Could you check a few things on this model? Use its own coordinates, in mm. Face numbers are marked on the shaded views. Give positions to 0.01 mm unless a question says otherwise; leave off trailing zeros. Order: outer loops, then holes, each group sorted by start corner. A loop starts at its lowest first (then second) coordinate and runs counter-clockwise, first axis right, second up. Notation, with made-up numbers: M 43.5,48.25 L 71.5,48.25 A29 cw 71.5,87.25 Z; hole C 63.25,24.25 d4. An arc over 180 degrees is marked long. Use a Markdown table: item, result. Add a question column.
```python
from build123d import *
from build123d.topology import SkipClean

# Parameters (mm, degrees)
SKETCH_1_R               = 18
EXTRUDE_1_DEPTH          = 1.5
EXTRUDE_2_DEPTH          = 6
EXTRUDE_2_DEPTH_BACK     = 6.5
SKETCH_2_R               = 20
SKETCH_2_R_2             = 18
CUT_EXTRUDE_START        = 1.5
SKETCH_6_R               = 1
CUT_EXTRUDE_4_DEPTH      = 8
CUT_EXTRUDE_5_DEPTH      = 30.393876913
CUT_EXTRUDE_5_DEPTH_BACK = 30.393876913
CUT_EXTRUDE_6_DEPTH      = 1.5
EXTRUDE_START            = 8
EXTRUDE_3_DEPTH          = 6.5
EXTRUDE_START_2          = 1.5
SKETCH_10_R              = 2.5
SKETCH_10_R_2            = 1.6
EXTRUDE_4_DEPTH          = 1.5


with BuildPart() as part:
    # 草图1 → 凸台-拉伸1 (new body)
    with BuildSketch(Plane(origin=(0, 0, 0), x_dir=(1, 0, 0), z_dir=(0, 1, 0))):
        with Locations(Location((0, 0, 0), (0, 0, 270))):
            Circle(SKETCH_1_R)
    extrude(amount=EXTRUDE_1_DEPTH)

    # 草图2 → 凸台-拉伸2 (add, two sides: drawn at the far end of the back side and taken through both)
    with BuildSketch(Plane(origin=(0, 0, 0), x_dir=(1, 0, 0), z_dir=(0, 1, 0)).offset(-EXTRUDE_2_DEPTH_BACK)):
        with Locations(Location((0, 0, 0), (0, 0, 270))):
            Circle(SKETCH_2_R)
        with Locations(Location((0, 0, 0), (0, 0, 270))):
            Circle(SKETCH_2_R_2, mode=Mode.SUBTRACT)
    extrude(amount=EXTRUDE_2_DEPTH + EXTRUDE_2_DEPTH_BACK)

    # 扫描2: sweep along a curve in space
    with SkipClean():  # the faces are left unmerged after this step: merging them gives an invalid solid
        with BuildLine() as sweep_2_path:
            ThreePointArc((0, 6, 18), (12.727922061, 6, 12.727922061), (18, 6, 0))
            ThreePointArc((18, 6, 0), (12.727922061, 6, -12.727922061), (0, 6, -18))
            ThreePointArc((0, 6, -18), (-12.727922061, 6, -12.727922061), (-18, 6, 0))
            ThreePointArc((-18, 6, 0), (-12.727922061, 6, 12.727922061), (0, 6, 18))
        # 草图5 → 扫描2 (sweep)
        with BuildSketch(Plane.XY):
            Polygon((-20, 6), (-18, 6), (-18, 8), align=None)
        sweep(path=sweep_2_path.line)

    # 草图6 → 切除-拉伸4 (cut)
    with SkipClean():  # the faces are left unmerged after this step: merging them gives an invalid solid
        with BuildSketch(Plane(origin=(0, 0, 0), x_dir=(1, 0, 0), z_dir=(0, 1, 0)).offset(CUT_EXTRUDE_START)):
            with Locations(Location((0, -12.5, 0), (0, 0, 270))):
                Circle(SKETCH_6_R)
            with Locations(Location((0, 12.5, 0), (0, 0, 270))):
                Circle(SKETCH_6_R)
        extrude(amount=-CUT_EXTRUDE_4_DEPTH, mode=Mode.SUBTRACT)

    # 草图7 → 切除-拉伸5 (cut, two sides: drawn at the far end of the back side and taken through both)
    with BuildSketch(Plane(origin=(0, 0, 0), x_dir=(1, 0, 0), z_dir=(0, 1, 0)).offset(-CUT_EXTRUDE_5_DEPTH_BACK)):
        with BuildLine():
            Line((-19.843134833, -2.5), (-15.07554347, -2.5))
            Line((-15.07554347, -2.5), (-15.07554347, 2.5))
            Line((-15.07554347, 2.5), (-19.843134833, 2.5))
            ThreePointArc((-19.843134833, 2.5), (-20, 0), (-19.843134833, -2.5))
        make_face()
        with BuildLine():
            Line((15.07554347, 2.5), (15.07554347, -2.5))
            Line((15.07554347, -2.5), (19.843134833, -2.5))
            ThreePointArc((19.843134833, -2.5), (20, 0), (19.843134833, 2.5))
            Line((19.843134833, 2.5), (15.07554347, 2.5))
        make_face()
    extrude(amount=CUT_EXTRUDE_5_DEPTH + CUT_EXTRUDE_5_DEPTH_BACK, mode=Mode.SUBTRACT)

    # 草图8 → 切除-拉伸6 (cut)
    with SkipClean():  # the faces are left unmerged after this step: merging them gives an invalid solid
        with BuildSketch(Plane(origin=(0, 0, 0), x_dir=(1, 0, 0), z_dir=(0, 1, 0)).offset(CUT_EXTRUDE_START)):
            with BuildLine():
                Line((10.606601706, 12.020815293), (12.001158233, 13.41537182))
                ThreePointArc((12.001158233, 13.41537182), (12.727922049, 12.727922074), (13.415371797, 12.001158259))
                Line((13.415371797, 12.001158259), (12.020815268, 10.606601731))
                ThreePointArc((12.020815268, 10.606601731), (10.606601706, 10.606601706), (10.606601706, 12.020815293))
            make_face()
            with BuildLine():
                Line((12.020815268, -10.606601731), (13.415371797, -12.001158259))
                ThreePointArc((13.415371797, -12.001158259), (12.727922049, -12.727922074), (12.001158233, -13.41537182))
                Line((12.001158233, -13.41537182), (10.606601706, -12.020815293))
                ThreePointArc((10.606601706, -12.020815293), (10.606601706, -10.606601706), (12.020815268, -10.606601731))
            make_face()
            with BuildLine():
                Line((-10.606601706, -12.020815293), (-12.001158233, -13.41537182))
                ThreePointArc((-12.001158233, -13.41537182), (-12.727922049, -12.727922074), (-13.415371797, -12.001158259))
                Line((-13.415371797, -12.001158259), (-12.020815268, -10.606601731))
                ThreePointArc((-12.020815268, -10.606601731), (-10.606601706, -10.606601706), (-10.606601706, -12.020815293))
            make_face()
            with BuildLine():
                Line((-12.020815268, 10.606601731), (-13.415371797, 12.001158259))
                ThreePointArc((-13.415371797, 12.001158259), (-12.727922049, 12.727922074), (-12.001158233, 13.41537182))
                Line((-12.001158233, 13.41537182), (-10.606601706, 12.020815293))
                ThreePointArc((-10.606601706, 12.020815293), (-10.606601706, 10.606601706), (-12.020815268, 10.606601731))
            make_face()
        extrude(amount=-CUT_EXTRUDE_6_DEPTH, mode=Mode.SUBTRACT)

    # 草图9 → 凸台-拉伸3 (add)
    with SkipClean():  # the faces are left unmerged after this step: merging them gives an invalid solid
        with BuildSketch(Plane(origin=(0, 0, 0), x_dir=(1, 0, 0), z_dir=(0, 1, 0)).offset(EXTRUDE_START)):
            with BuildLine():
                Line((12.020815268, -10.606601731), (13.415371797, -12.001158259))
                ThreePointArc((13.415371797, -12.001158259), (13.906042657, -11.428997228), (14.372329608, -10.836795727))
                Line((14.372329608, -10.836795727), (13.081475446, -9.545941553))
                ThreePointArc((13.081475446, -9.545941553), (9.545941558, -9.545941548), (9.545941537, -13.081475443))
                Line((9.545941537, -13.081475443), (10.8367957, -14.372329629))
                ThreePointArc((10.8367957, -14.372329629), (11.428997201, -13.906042679), (12.001158233, -13.41537182))
                Line((12.001158233, -13.41537182), (10.606601718, -12.020815281))
                ThreePointArc((10.606601718, -12.020815281), (10.606601731, -10.606601731), (12.020815268, -10.606601731))
            make_face()
            with BuildLine():
                Line((-10.606601718, -12.020815281), (-12.001158233, -13.41537182))
                ThreePointArc((-12.001158233, -13.41537182), (-11.428997201, -13.906042679), (-10.8367957, -14.372329629))
                Line((-10.8367957, -14.372329629), (-9.545941547, -13.081475453))
                ThreePointArc((-9.545941547, -13.081475453), (-9.545941551, -9.545941542), (-13.081475462, -9.545941556))
                Line((-13.081475462, -9.545941556), (-14.372329609, -10.836795726))
                ThreePointArc((-14.372329609, -10.836795726), (-13.906042657, -11.428997227), (-13.415371797, -12.001158259))
                Line((-13.415371797, -12.001158259), (-12.020815281, -10.606601718))
                ThreePointArc((-12.020815281, -10.606601718), (-10.606601718, -10.606601718), (-10.606601718, -12.020815281))
            make_face()
            with BuildLine():
                Line((10.606601718, 12.020815281), (12.001158233, 13.41537182))
                ThreePointArc((12.001158233, 13.41537182), (11.428997201, 13.906042679), (10.8367957, 14.372329629))
                Line((10.8367957, 14.372329629), (9.545941547, 13.081475453))
                ThreePointArc((9.545941547, 13.081475453), (9.545941551, 9.545941542), (13.081475462, 9.545941556))
                Line((13.081475462, 9.545941556), (14.372329609, 10.836795726))
                ThreePointArc((14.372329609, 10.836795726), (13.906042657, 11.428997227), (13.415371797, 12.001158259))
                Line((13.415371797, 12.001158259), (12.020815281, 10.606601718))
                ThreePointArc((12.020815281, 10.606601718), (10.606601718, 10.606601718), (10.606601718, 12.020815281))
            make_face()
            with BuildLine():
                Line((-12.020815268, 10.606601731), (-13.415371797, 12.001158259))
                ThreePointArc((-13.415371797, 12.001158259), (-13.906042657, 11.428997228), (-14.372329608, 10.836795727))
                Line((-14.372329608, 10.836795727), (-13.081475446, 9.545941553))
                ThreePointArc((-13.081475446, 9.545941553), (-9.545941558, 9.545941548), (-9.545941537, 13.081475443))
                Line((-9.545941537, 13.081475443), (-10.8367957, 14.372329629))
                ThreePointArc((-10.8367957, 14.372329629), (-11.428997201, 13.906042679), (-12.001158233, 13.41537182))
                Line((-12.001158233, 13.41537182), (-10.606601718, 12.020815281))
                ThreePointArc((-10.606601718, 12.020815281), (-10.606601731, 10.606601731), (-12.020815268, 10.606601731))
            make_face()
        extrude(amount=-EXTRUDE_3_DEPTH)

    # 草图10 → 凸台-拉伸4 (add)
    # profile 1 of 2: a face of its own
    with SkipClean():  # the faces are left unmerged after this step: merging them gives an invalid solid
        with BuildSketch(Plane(origin=(0, 0, 0), x_dir=(1, 0, 0), z_dir=(0, 1, 0)).offset(EXTRUDE_START_2)):
            with Locations(Location((0, 12.5, 0), (0, 0, 270))):
                Circle(SKETCH_10_R)
            with Locations(Location((0, 12.5, 0), (0, 0, 270))):
                Circle(SKETCH_10_R_2, mode=Mode.SUBTRACT)
        # profile 2 of 2: a face of its own
        with BuildSketch(Plane(origin=(0, 0, 0), x_dir=(1, 0, 0), z_dir=(0, 1, 0)).offset(EXTRUDE_START_2)):
            with Locations(Location((0, -12.5, 0), (0, 0, 270))):
                Circle(SKETCH_10_R)
            with Locations(Location((0, -12.5, 0), (0, 0, 270))):
                Circle(SKETCH_10_R_2, mode=Mode.SUBTRACT)
        extrude(amount=EXTRUDE_4_DEPTH)


solid = part.part
```
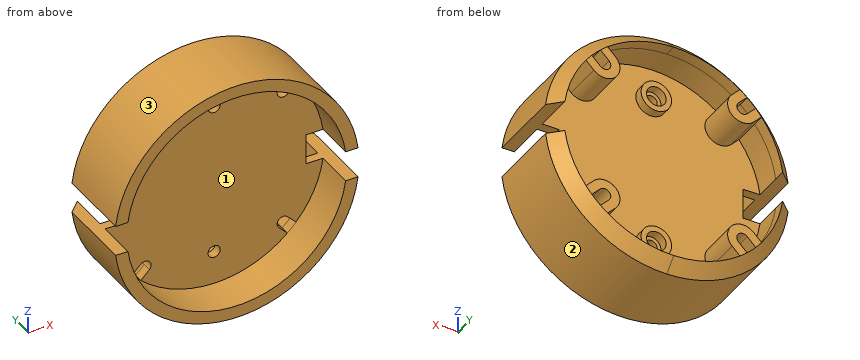
1) We'd pull the mould along Z, two halves only. Please class the marked faces 1, 2 and 3: pulls with the +Z half, pulls with the -Z half, needs draft (parallel to the pull), parting line crosses it, or undercut.
2) Suppose I cut it at C-C on z = -2. Please give me the cut outline in (x, y), and give its area (3 significant figures).
3) Please list where these lines run through material, in increasing order: line 1 (X direction, y = 2.6, z = -12.5); line 2 (Y direction, x = -7.5, z = 1); line 3 (X direction, y = 6.5, z = -8). Write a range as from..to.
4) Suppose I cut it at B-B on y = 5.5. Count the separate pieces of the cut face and the enclosed holes in it, and give its area (3 significant figures).
5) For pin 1 (10.5 mm diameter, centred on x = 1.5, z = -3, fed in from -Y); pin 2 (3 mm diameter, centred on x = 2.5, y = -2.5, fed in from -Z) (3 decimals); pin 3 (1.2 mm diameter, centred on y = 0.5, z = 0, fed in from -X), each with a flat end and sliding along its axis, tell me the tip position at first contact or that it passes through.
Values found:
| question | item | result |
|---|---|---|
| 1 | face 1 | undercut |
| 1 | face 2 | pulls with the -Z half |
| 1 | face 3 | pulls with the +Z half |
| 2 | outline | M -15.08,0 L 15.08,0 L 15.08,1.5 L -15.08,1.5 Z |
| 2 | area | 45.2 mm^2 |
| 3 | line 1 | x = -15.61..-12.95, -11.09..-9.11, -2.5..-1.6, 1.6..2.5, 9.11..11.09, 12.95..15.61 |
| 3 | line 2 | y = 0..1.5 |
| 3 | line 3 | x = -17.78..-16.12, 16.12..17.78 |
| 4 | separate pieces | 2 |
| 4 | enclosed holes | 4 |
| 4 | area | 275 mm^2 |
| 5 | pin 1 | stops at y = 0 |
| 5 | pin 2 | stops at z = -19.975 |
| 5 | pin 3 | stops at x = -15.08 |
